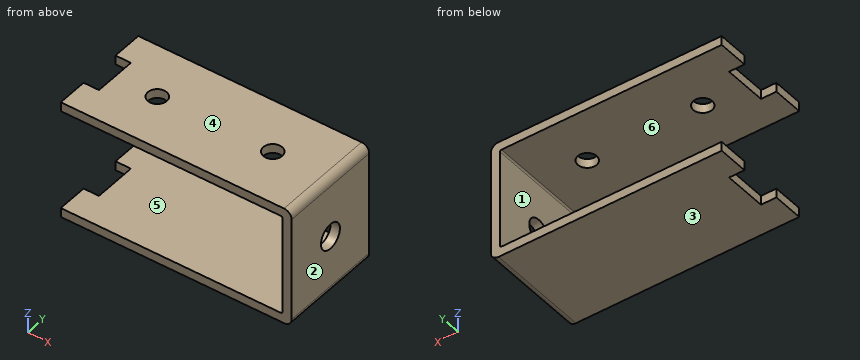
```python
from build123d import *

# Parameters (mm, degrees)
CROQUIS1_W                 = 30
CROQUIS1_H                 = 15.5
SALIENTE_EXTRUIR1_DEPTH    = 6.75
CROQUIS2_W                 = 28.8
CROQUIS2_H                 = 13.1
CORTAR_EXTRUIR1_DEPTH      = 7.75
CORTAR_EXTRUIR1_DEPTH_BACK = 7.75
CORTAR_EXTRUIR2_REACH      = 32
CROQUIS3_R                 = 1.65
REDONDEO1_R                = 1
REDONDEO2_R                = 0.2
CROQUIS4_W                 = 2
CROQUIS4_H                 = 5.55
CORTAR_EXTRUIR3_DEPTH      = 8.75
CORTAR_EXTRUIR3_DEPTH_BACK = 8.75
CORTAR_EXTRUIR4_REACH      = 17.5
CROQUIS5_R                 = 1.225


with BuildPart() as part:
    # Croquis1 → Saliente-Extruir1 (new body, symmetric)
    with BuildSketch(Plane(origin=(0, 0, 0), x_dir=(1, 0, 0), z_dir=(0, 1, 0))):
        Rectangle(CROQUIS1_W, CROQUIS1_H)
    extrude(amount=SALIENTE_EXTRUIR1_DEPTH, both=True)

    # Croquis2 → Cortar-Extruir1 (cut, two sides)
    with BuildSketch(Plane(origin=(0, 0, 0), x_dir=(1, 0, 0), z_dir=(0, 1, 0))) as cortar_extruir1_sk:
        with Locations((-0.6, 0)):
            Rectangle(CROQUIS2_W, CROQUIS2_H)
    extrude(amount=CORTAR_EXTRUIR1_DEPTH, mode=Mode.SUBTRACT)
    extrude(cortar_extruir1_sk.sketch, amount=-CORTAR_EXTRUIR1_DEPTH_BACK, mode=Mode.SUBTRACT)

    # Croquis3 → Cortar-Extruir2 (cut, up to next)
    with BuildSketch(Plane(origin=(15, 0, 0), x_dir=(0, 0, -1), z_dir=(1, 0, 0)), mode=Mode.PRIVATE) as cortar_extruir2_sk1:
        Circle(CROQUIS3_R)
    cortar_extruir2_tool1 = extrude(cortar_extruir2_sk1.sketch, amount=-CORTAR_EXTRUIR2_REACH, mode=Mode.PRIVATE) & part.part
    add(cortar_extruir2_tool1.solids().sort_by_distance((15, 0, 0))[0], mode=Mode.SUBTRACT)

    # Redondeo1
    redondeo1_edges = [part.edges().sort_by_distance(p)[0] for p in [
        (15, 0, -7.75),
        (15, 0, 7.75),
    ]]
    fillet(redondeo1_edges, radius=REDONDEO1_R)

    # Redondeo2
    redondeo2_edges = [part.edges().sort_by_distance(p)[0] for p in [
        (13.8, 0, -6.55),
        (13.8, 0, 6.55),
    ]]
    fillet(redondeo2_edges, radius=REDONDEO2_R)

    # Croquis4 → Cortar-Extruir3 (cut, two sides)
    with BuildSketch(Plane.XY) as cortar_extruir3_sk:
        with Locations((-14, 0)):
            Rectangle(CROQUIS4_W, CROQUIS4_H)
    extrude(amount=CORTAR_EXTRUIR3_DEPTH, mode=Mode.SUBTRACT)
    extrude(cortar_extruir3_sk.sketch, amount=-CORTAR_EXTRUIR3_DEPTH_BACK, mode=Mode.SUBTRACT)

    # Croquis5 → Cortar-Extruir4 (cut, up to next)
    with BuildSketch(Plane.XY.offset(7.75), mode=Mode.PRIVATE) as cortar_extruir4_sk1:
        with Locations((-7.5, 0)):
            Circle(CROQUIS5_R)
    cortar_extruir4_tool1 = extrude(cortar_extruir4_sk1.sketch, amount=-CORTAR_EXTRUIR4_REACH, mode=Mode.PRIVATE) & part.part
    add(cortar_extruir4_tool1.solids().sort_by_distance((-7.5, 0, 7.75))[0], mode=Mode.SUBTRACT)
    # Croquis5 → Cortar-Extruir4 (cut, up to next)
    with BuildSketch(Plane.XY.offset(7.75), mode=Mode.PRIVATE) as cortar_extruir4_sk2:
        with Locations((7.5, 0)):
            Circle(CROQUIS5_R)
    cortar_extruir4_tool2 = extrude(cortar_extruir4_sk2.sketch, amount=-CORTAR_EXTRUIR4_REACH, mode=Mode.PRIVATE) & part.part
    add(cortar_extruir4_tool2.solids().sort_by_distance((7.5, 0, 7.75))[0], mode=Mode.SUBTRACT)


solid = part.part
```
Design review of the part built by this model. Coordinates are the model's own, in mm. Face numbers are marked on the shaded views. A direction names the side the tool comes from. Give positions to 0.01 mm unless a question says otherwise; leave off trailing zeros. Write each loop counter-clockwise with the first axis right and the second up, starting at its lowest first coordinate (ties: lowest second). Pieces come first, ordered by that corner, then holes. Notation, with made-up numbers: (-19, 41) -> (-10, 41) arc R17 cw to (-10, 60) -> close; hole circle Ø6 at (1.5, 0.5). An arc over 180 degrees is marked (long way). Answer in a Markdown table with one row per item.
(1) Consider section D-D (y = -2.25). State the section outline as (x, z) points, then the cut area to 3 significant figures.
Results:
| item | result |
|---|---|
| outline | (-13, -7.75) -> (14, -7.75) arc R1 ccw to (15, -6.75) -> (15, 6.75) arc R1 ccw to (14, 7.75) -> (-13, 7.75) -> (-13, 6.55) -> (13.6, 6.55) arc R0.2 cw to (13.8, 6.35) -> (13.8, -6.35) arc R0.2 cw to (13.6, -6.55) -> (-13, -6.55) -> close |
| area | 82.5 mm2 |
(2) Clearance check with flat-ended pins moving along their axes: pin 1 (4 mm diameter, centred on y = 2, z = 3, fed in from -X); pin 2 (8 mm diameter, centred on x = 8.5, z = 2.5, fed in from -Y). State where each tip first meets the part, or that it passes through.
Results:
| item | result |
|---|---|
| pin 1 | x = 13.8 |
| pin 2 | through |
(3) To check wall thickness, follow probe 1 along Z at (x, y) = (3.25, 3); probe 2 along Y at (x, z) = (14.45, 0); probe 3 along Y at (x, z) = (-13.5, 6.75) (3 decimals). State the ranges of each line that lie inside material, in increasing order.
Results:
| item | result |
|---|---|
| probe 1 | -7.75 to -6.55, 6.55 to 7.75 |
| probe 2 | -6.75 to -1.65, 1.65 to 6.75 |
| probe 3 | -6.75 to -2.775, 2.775 to 6.75 |
(4) Consider section A-A (z = 0). State the section outline as (x, y) points.
Results:
| item | result |
|---|---|
| outline | (13.8, -6.75) -> (15, -6.75) -> (15, -1.65) -> (13.8, -1.65) -> close; (13.8, 1.65) -> (15, 1.65) -> (15, 6.75) -> (13.8, 6.75) -> close |
(5) For the marked faces 1 and 2, list the 3-axis set-ups (+Z, -Z, +X, -X, +Y, -Y) from which the entire face can be reached by the end or side of a thin tool; tool diameter is ignored.
Results:
| item | result |
|---|---|
| face 1 | -X, +Y, -Y |
| face 2 | +Z, -Z, +X, +Y, -Y |
(6) Consider section B-B (x = 7.5). State the section outline as (y, z) points (3 decimals).
Results:
| item | result |
|---|---|
| outline | (-6.75, -7.75) -> (6.75, -7.75) -> (6.75, -6.55) -> (-6.75, -6.55) -> close; (-6.75, 6.55) -> (-1.225, 6.55) -> (-1.225, 7.75) -> (-6.75, 7.75) -> close; (1.225, 6.55) -> (6.75, 6.55) -> (6.75, 7.75) -> (1.225, 7.75) -> close |
(7) Mouldability with a two-part tool opening along Z and no side actions: class the marked faces 3, 4, 5 and 6 as +Z half, -Z half, draft (parallel to the pull), parting line (faces both ways), or undercut.
Results:
| item | result |
|---|---|
| face 3 | -Z half |
| face 4 | +Z half |
| face 5 | undercut |
| face 6 | undercut |
(8) Consider section C-C (y = 0). State the section outline as (x, z) points (3 decimals).
Results:
| item | result |
|---|---|
| outline | (-13, -7.75) -> (14, -7.75) arc R1 ccw to (15, -6.75) -> (15, -1.65) -> (13.8, -1.65) -> (13.8, -6.35) arc R0.2 cw to (13.6, -6.55) -> (-13, -6.55) -> close; (-13, 6.55) -> (-8.725, 6.55) -> (-8.725, 7.75) -> (-13, 7.75) -> close; (-6.275, 6.55) -> (6.275, 6.55) -> (6.275, 7.75) -> (-6.275, 7.75) -> close; (8.725, 6.55) -> (13.6, 6.55) arc R0.2 cw to (13.8, 6.35) -> (13.8, 1.65) -> (15, 1.65) -> (15, 6.75) arc R1 ccw to (14, 7.75) -> (8.725, 7.75) -> close |
